Here's how the part is built. I have some questions about the finished solid (model axes, mm). A direction names the side the tool comes from. Coordinates: 2 decimals unless noted, no trailing zeros. Write each loop counter-clockwise with the first axis right and the second up, starting at its lowest first coordinate (ties: lowest second). Pieces come first, ordered by that corner, then holes.
from build123d import *

# Parameters (mm, degrees)
PAD_DEPTH    = 0.5
SKETCH_R     = 1.5
PAD001_DEPTH = 1.5


with BuildPart() as part:
    # Sketch002 → Pad (new body)
    with BuildSketch(Plane.XY.offset(1.4)):
        Polygon((-7.5, 5), (7.5, 5), (7.5, -5), (-6, -5), (-7.5, -3.5), align=None)
    extrude(amount=PAD_DEPTH)

    # Sketch (on Face6 of Pad) → Pad001 (join)
    with BuildSketch(Plane(origin=(0, 0, 1.4), x_dir=(1, 0, 0), z_dir=(0, 0, -1))):
        Circle(SKETCH_R)
    extrude(amount=PAD001_DEPTH)


solid = part.part
1. I want a section at A-A (x = 0). List the corners of the cut face in (y, z) for me, then the cut area to 3 significant figures.
2. If I drill on line 1 (Z direction, x = -1, y = 4.75); line 2 (X direction, y = 1.25, z = 0.5); line 3 (X direction, y = -0.5, z = 0.15), over which ranges is the centre line in solid material (lowest first)?
3. On a 3-axis mill with a long thin cutter (end or side, diameter ignored), from which of +Z, -Z, +X, -X, +Y, -Y can I reach the whole of each face in a straight line? I mean faces 1 (the face through (-6.7, -4.3, 1.6)), 2 (the face through (-1.5, -0.07, 0.66)). Say none if no direction works.
4. For pin 1 Ø3 at (x, y) = (-4.5, -2) entering from -Z; pin 2 Ø6 at (x, y) = (3.5, 1.5) entering from -Z, each with a flat end and sliding along its axis, tell me the tip position at first contact or that it passes through.
5. I want a section at C-C (z = 0.5). List the corners of the cut face in (x, y) for me, then the cut area to 3 significant figures.
6. I want a section at D-D (y = -3.75). List the corners of the cut face in (x, z) for me, then the cut area to 4 significant figures.
7. I want a section at B-B (y = 0). List the corners of the cut face in (x, z) for me.
Response values:
1. outline: (-5, 1.4) - (-1.5, 1.4) - (-1.5, -0.1) - (1.5, -0.1) - (1.5, 1.4) - (5, 1.4) - (5, 1.9) - (-5, 1.9) - close
1. area: 9.50 mm2
2. line 1: z = 1.4 to 1.9
2. line 2: x = -0.83 to 0.83
2. line 3: x = -1.41 to 1.41
3. face 1: +Z, -Z, -X, -Y
3. face 2: -Z
4. pin 1: stops at z = 1.4
4. pin 2: stops at z = -0.1
5. outline: circle Ø3 at (0, 0)
5. area: 7.07 mm2
6. outline: (-7.25, 1.4) - (7.5, 1.4) - (7.5, 1.9) - (-7.25, 1.9) - close
6. area: 7.375 mm2
7. outline: (-7.5, 1.4) - (-1.5, 1.4) - (-1.5, -0.1) - (1.5, -0.1) - (1.5, 1.4) - (7.5, 1.4) - (7.5, 1.9) - (-7.5, 1.9) - close
